Can you work these out from the model? Positions are in its coordinate system, mm. Give positions to 0.01 mm unless a question says otherwise; leave off trailing zeros. Order: outer loops, then holes, each group sorted by start corner. A loop starts at its lowest first (then second) coordinate and runs counter-clockwise, first axis right, second up. Notation, with made-up numbers: M -35,89 L 14,89 A30 ccw 14,114 Z; hole C -5.5,30 d3. An arc over 180 degrees is marked long. Answer as a JSON object with one key per item and string values.
```python
from build123d import *

# Parameters (mm, degrees)
F0_W     = 330.2
F0_H     = 101.6
F1_DEPTH = 19.05


with BuildPart() as f1:
    # F0 (on Front) → F1 (new body)
    with BuildSketch(Plane.XZ):
        with Locations((-165.1, 50.8)):
            Rectangle(F0_W, F0_H)
        Polygon((-311.15, 33.914647), (-311.15, 46.614647), (-311.15, 59.314647), (-292.1, 59.314647), (-292.1, 46.614647), (-292.1, 33.914647), align=None, mode=Mode.SUBTRACT)
        Polygon((-38.1, 33.914647), (-38.1, 46.614647), (-38.1, 59.314647), (-19.05, 59.314647), (-19.05, 46.614647), (-19.05, 33.914647), align=None, mode=Mode.SUBTRACT)
    extrude(amount=F1_DEPTH)


solid = f1.part
```
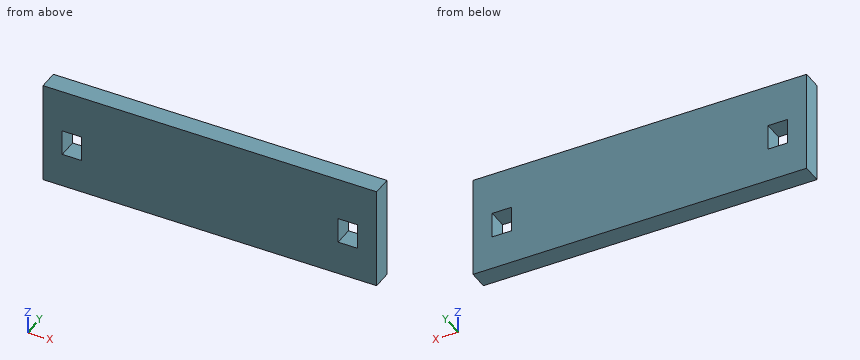
1) I want a section at B-B on x = -28. Write out the boundary of the cut face in (y, z), and give its area (3 significant figures).
Results found:
{"outline": "M -19.05,0 L 0,0 L 0,33.91 L -19.05,33.91 Z; M -19.05,59.31 L 0,59.31 L 0,101.6 L -19.05,101.6 Z", "area": "1,450 mm²"}
2) I need wall thicknesses on L1, parallel to X at y = -16.5, z = 58; L2, parallel to Z at x = -25, y = -4. Which ranges of each line are inside material? Lowest first, please.
Results found:
{"L1": "x = -330.2 to -311.15, -292.1 to -38.1, -19.05 to 0", "L2": "z = 0 to 33.91, 59.31 to 101.6"}
3) I want a section at C-C on z = 44. Write out the boundary of the cut face in (x, y).
Results found:
{"outline": "M -330.2,-19.05 L -311.15,-19.05 L -311.15,0 L -330.2,0 Z; M -292.1,-19.05 L -38.1,-19.05 L -38.1,0 L -292.1,0 Z; M -19.05,-19.05 L 0,-19.05 L 0,0 L -19.05,0 Z"}
4) I want a section at A-A on y = -7.75. Write out the boundary of the cut face in (x, z).
Results found:
{"outline": "M -330.2,0 L 0,0 L 0,101.6 L -330.2,101.6 Z; hole M -311.15,33.91 L -292.1,33.91 L -292.1,59.31 L -311.15,59.31 Z; hole M -38.1,33.91 L -19.05,33.91 L -19.05,59.31 L -38.1,59.31 Z"}
